Build history of the part. All positions in model axes, mm. Coordinates: 2 decimals unless noted, no trailing zeros. Order: outer loops, then holes, each group sorted by start corner. A loop starts at its lowest first (then second) coordinate and runs counter-clockwise, first axis right, second up. Notation, with made-up numbers: (49, 8) - (105, 8) arc R11 ccw to (105, 20) - close; hole circle Ø8 at (54, -31.5). An arc over 180 degrees is marked (long way). Return JSON: item names as keys, results as strings.
from build123d import *

# Parameters (mm, degrees)
SKETCH_1_R          = 70
EXTRUDE_1_DEPTH     = 90
SKETCH_2_R          = 38
CUT_EXTRUDE_1_DEPTH = 134.790881603
CUT_EXTRUDE_START   = -45
SKETCH_3_R          = 70
SKETCH_3_R_2        = 45
CUT_EXTRUDE_2_DEPTH = 45
FILLET_1_R          = 2


with BuildPart() as part:
    # 草图1 → 凸台-拉伸1 (new body)
    with BuildSketch(Plane.XY):
        with Locations(Location((0, 0, 0), (0, 0, 180))):
            Circle(SKETCH_1_R)
    extrude(amount=EXTRUDE_1_DEPTH)

    # 草图2 → 切除-拉伸1 (cut, through all)
    with BuildSketch(Plane.XY.offset(90)):
        Circle(SKETCH_2_R)
    extrude(amount=-CUT_EXTRUDE_1_DEPTH, mode=Mode.SUBTRACT)

    # 草图3 → 切除-拉伸2 (cut)
    with BuildSketch(Plane.XY.offset(90).offset(CUT_EXTRUDE_START)):
        with Locations(Location((0, 0, 0), (0, 0, 180))):
            Circle(SKETCH_3_R)
        Circle(SKETCH_3_R_2, mode=Mode.SUBTRACT)
    extrude(amount=CUT_EXTRUDE_2_DEPTH, mode=Mode.SUBTRACT)

    # 圆角1
    fillet_1_edges = [part.edges().sort_by_distance(p)[0] for p in [
        (-45, 0, 90),
        (70, 0, 0),
    ]]
    fillet(fillet_1_edges, radius=FILLET_1_R)


solid = part.part
1. Probe L1, parallel to Y at x = 0, z = 28.5; L2, parallel to Z at x = -47, y = -34; L3, parallel to Y at x = 0, z = 53.5. List the from-to ranges inside material, lowest first.
Check values:
{"L1": "-70 to -38, 38 to 70", "L2": "0 to 45", "L3": "-45 to -38, 38 to 45"}
2. Drop flat-ended pins along their axis: pin 1 (1 mm diameter, centred on y = 44, z = 40, fed in from +X); pin 2 (8 mm diameter, centred on y = -55.5, z = 10.5, fed in from +X); pin 3 (12 mm diameter, centred on y = 19.5, z = 10, fed in from -X). Give the stop position or say it passes through.
Check values:
{"pin 1": "x = 54.84", "pin 2": "x = 47.41", "pin 3": "x = -68.69"}
3. Mould opens along Y. For faces 1 (the cylindrical face through (20.765, -39.923, 66.199)), 2 (the cylindrical face through (17.535, -33.713, 45.63)), 3 (the flat face through (1, 46, 45)) say: pulls with the +Y half, pulls with the -Y half, needs draft (parallel to the pull), parting line crosses it, or undercut.
Check values:
{"face 1": "parting line crosses it", "face 2": "undercut", "face 3": "needs draft"}
4. Cut at A-A on x = 0. Give the cut face in (y, z), plus the area to 3 significant figures.
Check values:
{"outline": "(-70, 2) arc R2 ccw to (-68, 0) - (-38, 0) - (-38, 90) - (-43, 90) arc R2 ccw to (-45, 88) - (-45, 45) - (-70, 45) - close; (38, 0) - (68, 0) arc R2 ccw to (70, 2) - (70, 45) - (45, 45) - (45, 88) arc R2 ccw to (43, 90) - (38, 90) - close", "area": "3,510 mm²"}
